```python
from build123d import *

# Parameters (mm, degrees)
ESQUISSE1_W        = 180
ESQUISSE1_H        = 300
ESQUISSE1_W_2      = 55
ESQUISSE1_H_2      = 130
BOSS_EXTRU_1_DEPTH = 6.35


with BuildPart() as part:
    # Esquisse1 → Boss.-Extru.1 (new body)
    with BuildSketch(Plane(origin=(0, 0, 0), x_dir=(1, 0, 0), z_dir=(0, 1, 0))):
        Rectangle(ESQUISSE1_W, ESQUISSE1_H)
        with Locations((-117.5, 0)):
            Rectangle(ESQUISSE1_W_2, ESQUISSE1_H_2)
        with Locations((117.5, 0)):
            Rectangle(ESQUISSE1_W_2, ESQUISSE1_H_2)
        with BuildLine():
            Line((-90, -150), (90, -150))
            ThreePointArc((90, -150), (0, -165), (-90, -150))
        make_face()
        with BuildLine():
            ThreePointArc((-90, 150), (0, 165), (90, 150))
            Line((90, 150), (-90, 150))
        make_face()
    extrude(amount=BOSS_EXTRU_1_DEPTH)


solid = part.part
```
For this review, take the finished solid that the model builds, in its own axes (mm). Give positions to 0.01 mm unless a question says otherwise; leave off trailing zeros. Loops run counter-clockwise (first coordinate to the right, second up) from the corner with the lowest first, then second, coordinate; pieces in that order, holes last. Notation, with made-up numbers: M -15,3.25 L 0,3.25 A22 ccw 0,26.25 Z; hole C -28,20 d9. An arc over 180 degrees is marked long. One line per item, written item: value. Start each with the question number.
Q1. Add section C-C (x = 125.5). Give the boundary of the cut face in (y, z).
Q2. Clearance check with flat-ended pins moving along their axes: pin 1 Ø1.5 at (x, y) = (35, 4) entering from +Z; pin 2 Ø3 at (y, z) = (3, 99) entering from -X; pin 3 Ø1.9 at (y, z) = (2.5, -120.5) entering from +X. State where each tip first meets the part, or that it passes through.
Q3. Add section A-A (y = 3). Give the boundary of the cut face in (x, z), and give its area (3 significant figures).
Q4. Add section B-B (z = 121). Give the boundary of the cut face in (x, y).
Q5. For L1, parallel to Z at x = -128, y = 6; L2, parallel to X at y = 6.25, z = -144.5; L3, parallel to Z at x = -67.5, y = 3, list the stretches that pass through material, from the lowest coordinate up.
Reply:
1. outline: M 0,-65 L 6.35,-65 L 6.35,65 L 0,65 Z
2. pin 1: z = 162.88
2. pin 2: x = -90
2. pin 3: x = 90
3. outline: M -145,-65 L -90,-65 L -90,-150 A277.5 ccw 90,-150 L 90,-65 L 145,-65 L 145,65 L 90,65 L 90,150 A277.5 ccw -90,150 L -90,65 L -145,65 Z
3. area: 71,900 mm²
4. outline: M -90,0 L 90,0 L 90,6.35 L -90,6.35 Z
5. L1: -65 to 65
5. L2: -90 to 90
5. L3: -156.67 to 156.67
